The figure shows three views and two pictorial views of one solid part (mm, origin at its lowest corner). Answer the questions. A direction names the side the tool comes from. Give positions to 0.01 mm unless a question says otherwise; leave off trailing zeros. Order: outer loops, then holes, each group sorted by start corner. A loop starts at its lowest first (then second) coordinate and runs counter-clockwise, first axis right, second up. Notation, with made-up numbers: M 65,-37.75 L 74,-37.75 A5 cw 74,-29.75 Z; hole C 13.25,38 d3. An arc over 180 degrees is marked long. One line per item, written item: value.
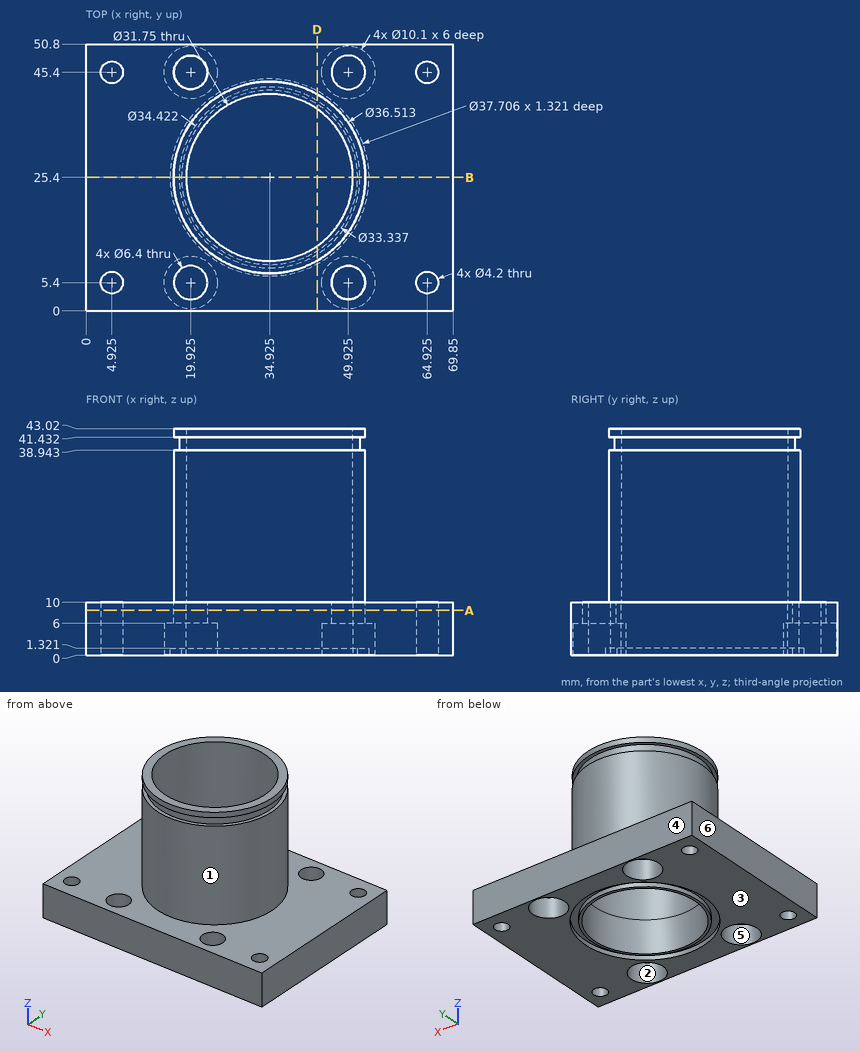
1) Determine the mould class of the marked faces 4, 5 and 6 for opening direction X: +X half, -X half, draft (parallel to the pull), parting line (faces both ways), or undercut.
Reported:
face 4: draft
face 5: undercut
face 6: -X half
2) Find section A-A, the plane z = 8.5. Count the separate pieces of the cut face and the enclosed holes in it, plus the area to 3 significant figures.
Reported:
separate pieces: 1
enclosed holes: 9
area: 2,570 mm^2
3) Which of the six approach directions +Z, -Z, +X, -X, +Y, -Y give full straight-line access (tool end or side, diameter ignored) to the marked faces 1, 2 and 3?
Reported:
face 1: +Z
face 2: -Z
face 3: -Z, +X, -X, +Y, -Y
4) Consider probe 1 along Z at (x, y) = (60.5, 44.5); probe 2 along Y at (x, z) = (35.5, 14.5) (1 decimal); probe 3 along Y at (x, z) = (65.5, 7). Determine where each line is inside the solid, lowest interval first.
Reported:
probe 1: z = 0 to 10
probe 2: y = 7.2 to 9.5, 41.3 to 43.6
probe 3: y = 0 to 3.38, 7.42 to 43.38, 47.42 to 50.8
5) Find section B-B, the plane y = 25.4. Write down the section's boundary in (x, z).
Reported:
outline: M 0,0 L 16.07,0 L 16.07,1.32 L 18.26,1.32 L 18.26,0 L 19.05,0 L 19.05,43.02 L 16.67,43.02 L 16.67,41.43 L 17.71,41.43 L 17.71,38.94 L 16.67,38.94 L 16.67,10 L 0,10 Z; M 50.8,0 L 51.59,0 L 51.59,1.32 L 53.78,1.32 L 53.78,0 L 69.85,0 L 69.85,10 L 53.18,10 L 53.18,38.94 L 52.14,38.94 L 52.14,41.43 L 53.18,41.43 L 53.18,43.02 L 50.8,43.02 Z
6) Find section D-D, the plane x = 44. Write down the section's boundary in (y, z) (1 decimal).
Reported:
outline: M 0,0 L 8.9,0 L 8.9,1.3 L 11.4,1.3 L 11.4,0 L 12.4,0 L 12.4,43 L 9.6,43 L 9.6,41.4 L 10.8,41.4 L 10.8,38.9 L 9.6,38.9 L 9.6,10 L 0,10 Z; M 38.4,0 L 39.4,0 L 39.4,1.3 L 41.9,1.3 L 41.9,0 L 50.8,0 L 50.8,10 L 41.2,10 L 41.2,38.9 L 40,38.9 L 40,41.4 L 41.2,41.4 L 41.2,43 L 38.4,43 Z
7) Each of these flat-tipped pins is pushed along its axis until it touches: pin 1 Ø3 at (x, y) = (58.5, 42) entering from +Z; pin 2 Ø8 at (x, y) = (49.925, 45.4) entering from -Z; pin 3 Ø6 at (x, y) = (19.925, 45.4) entering from -Z; pin 4 Ø3 at (y, z) = (35.5, 24.5) entering from +X. Where does it stop, or does it pass through?
Reported:
pin 1: stops at z = 10
pin 2: stops at z = 6
pin 3: passes through
pin 4: stops at x = 51.03
